```python
from build123d import *

# Parameters (mm, degrees)
SKETCH_W        = 142
SKETCH_H        = 67
PAD_DEPTH       = 25
THICKNESS_T     = 2.5
SKETCH001_R     = 4.3
SKETCH001_R_2   = 1.8
PAD001_DEPTH    = 5.5
FILLET_R        = 1
SKETCH002_W     = 32
SKETCH002_H     = 18.6
POCKET_DEPTH    = 5
SKETCH003_W     = 52
SKETCH003_H     = 20
POCKET001_DEPTH = 2.5
SKETCH006_R     = 1.8
POCKET002_DEPTH = 27.501
PAD005_DEPTH    = 2.5
FILLET001_R     = 2
CHAMFER001_SIZE = 1.2
FILLET002_R     = 2
CHAMFER002_SIZE = 1.2
POCKET003_DEPTH = 3
CHAMFER003_SIZE = 0.7


with BuildPart() as part:
    # Sketch → Pad (new body)
    with BuildSketch(Plane.XY):
        Rectangle(SKETCH_W, SKETCH_H)
    extrude(amount=PAD_DEPTH)

    # Thickness
    thickness_openings = [part.faces().sort_by_distance(p)[0] for p in [
        (0, 0, 25),
    ]]
    offset(amount=THICKNESS_T, openings=thickness_openings)

    # Sketch001 (on Face5 of Thickness) → Pad001 (join)
    with BuildSketch(Plane.XY):
        with Locations((-65, -27.5)):
            Circle(SKETCH001_R)
        with Locations((-65, -27.5)):
            Circle(SKETCH001_R_2, mode=Mode.SUBTRACT)
        with Locations((-65, 27.5)):
            Circle(SKETCH001_R)
        with Locations((-65, 27.5)):
            Circle(SKETCH001_R_2, mode=Mode.SUBTRACT)
        with Locations((-20, 27.5)):
            Circle(SKETCH001_R)
        with Locations((-20, 27.5)):
            Circle(SKETCH001_R_2, mode=Mode.SUBTRACT)
        with Locations((65, 27.5)):
            Circle(SKETCH001_R)
        with Locations((65, 27.5)):
            Circle(SKETCH001_R_2, mode=Mode.SUBTRACT)
        with Locations((65, -27.5)):
            Circle(SKETCH001_R)
        with Locations((65, -27.5)):
            Circle(SKETCH001_R_2, mode=Mode.SUBTRACT)
    extrude(amount=PAD001_DEPTH)

    # Fillet
    fillet_edges = [part.edges().sort_by_distance(p)[0] for p in [
        (-71, 33.5, 12.5),
        (71, 33.5, 12.5),
        (-71, -33.5, 12.5),
        (71, -33.5, 12.5),
    ]]
    fillet(fillet_edges, radius=FILLET_R)

    # Sketch002 (on Face19 of Fillet) → Pocket (cut)
    with BuildSketch(Plane(origin=(0, 36, 0), x_dir=(-1, 0, 0), z_dir=(0, 1, 0))):
        with Locations((-5.2475, 15.7)):
            Rectangle(SKETCH002_W, SKETCH002_H)
        with Locations((43.65, 15.7)):
            Rectangle(SKETCH002_W, SKETCH002_H)
        with BuildLine():
            ThreePointArc((-42.45, 25), (-47.8, 30.35), (-53.15, 25))
            Line((-53.15, 25), (-53.15, 9.6))
            ThreePointArc((-53.15, 9.6), (-47.8, 4.25), (-42.45, 9.6))
            Line((-42.45, 25), (-42.45, 9.6))
        make_face()
        with BuildLine():
            ThreePointArc((-25.95, 25), (-31.3, 30.35), (-36.65, 25))
            Line((-36.65, 25), (-36.65, 9.6))
            ThreePointArc((-36.65, 9.6), (-31.3, 4.25), (-25.95, 9.6))
            Line((-25.95, 25), (-25.95, 9.6))
        make_face()
    extrude(amount=-POCKET_DEPTH, mode=Mode.SUBTRACT)

    # Sketch003 (on Face35 of Pocket) → Pocket001 (cut)
    with BuildSketch(Plane.XZ.offset(36)):
        with Locations((-1.1, 15)):
            Rectangle(SKETCH003_W, SKETCH003_H)
    extrude(amount=-POCKET001_DEPTH, mode=Mode.SUBTRACT)

    # Sketch006 (on Face61 of Pocket001) → Pocket002 (cut, through all)
    with BuildSketch(Plane(origin=(0, 0, -2.5), x_dir=(1, 0, 0), z_dir=(0, 0, -1))):
        with Locations((-65, 27.5)):
            Circle(SKETCH006_R)
        with Locations((65, 27.5)):
            Circle(SKETCH006_R)
        with Locations((65, -27.5)):
            Circle(SKETCH006_R)
        with Locations((-20, -27.5)):
            Circle(SKETCH006_R)
        with Locations((-65, -27.5)):
            Circle(SKETCH006_R)
    extrude(amount=-POCKET002_DEPTH, mode=Mode.SUBTRACT)

    # Sketch008 (on Face32 of Pocket002) → Pad005 (join)
    with BuildSketch(Plane(origin=(0, 36, 0), x_dir=(-1, 0, 0), z_dir=(0, 1, 0))):
        with BuildLine():
            ThreePointArc((-42.45, 9.6), (-47.8, 14.95), (-53.15, 9.6))
            Line((-53.15, 9.6), (-53.15, 25))
            Line((-53.15, 25), (-42.45, 25))
            Line((-42.45, 25), (-42.45, 9.6))
        make_face()
        with BuildLine():
            ThreePointArc((-25.95, 9.6), (-31.3, 14.95), (-36.65, 9.6))
            Line((-36.65, 9.6), (-36.65, 25))
            Line((-36.65, 25), (-25.95, 25))
            Line((-25.95, 25), (-25.95, 9.6))
        make_face()
    extrude(amount=-PAD005_DEPTH)

    # Fillet001
    fillet001_edges = [part.edges().sort_by_distance(p)[0] for p in [
        (21.2475, 34.75, 6.4),
        (-10.7525, 34.75, 6.4),
        (-27.65, 34.75, 6.4),
        (-59.65, 34.75, 6.4),
    ]]
    fillet(fillet001_edges, radius=FILLET001_R)

    # Chamfer001
    chamfer001_edges = [part.edges().sort_by_distance(p)[0] for p in [
        (31.3, 36, 4.25),
        (47.8, 36, 4.25),
        (5.2475, 36, 6.4),
        (-43.65, 36, 6.4),
    ]]
    chamfer(chamfer001_edges, length=CHAMFER001_SIZE)

    # Fillet002
    fillet002_edges = [part.edges().sort_by_distance(p)[0] for p in [
        (24.9, -34.75, 5),
        (-27.1, -34.75, 5),
    ]]
    fillet(fillet002_edges, radius=FILLET002_R)

    # Chamfer002
    chamfer002_edges = [part.edges().sort_by_distance(p)[0] for p in [
        (-1.1, -36, 5),
    ]]
    chamfer(chamfer002_edges, length=CHAMFER002_SIZE)

    # Sketch010 (on Face14 of Chamfer002) → Pocket003 (cut)
    with BuildSketch(Plane.XY.offset(25)):
        with BuildLine():
            Line((-70, 33.7), (70, 33.7))
            ThreePointArc((71.2, 32.5), (70.848528, 33.348528), (70, 33.7))
            Line((71.2, 32.5), (71.2, -32.5))
            ThreePointArc((70, -33.7), (70.848528, -33.348528), (71.2, -32.5))
            Line((70, -33.7), (-70, -33.7))
            ThreePointArc((-71.2, -32.5), (-70.848528, -33.348528), (-70, -33.7))
            Line((-71.2, -32.5), (-71.2, 32.5))
            ThreePointArc((-70, 33.7), (-70.848528, 33.348528), (-71.2, 32.5))
        make_face()
    extrude(amount=-POCKET003_DEPTH, mode=Mode.SUBTRACT)

    # Chamfer003
    chamfer003_edges = [part.edges().sort_by_distance(p)[0] for p in [
        (-65.925, 36, 25),
        (-19.20125, 36, 25),
        (31.3, 36, 25),
    ]]
    chamfer(chamfer003_edges, length=CHAMFER003_SIZE)


solid = part.part
```
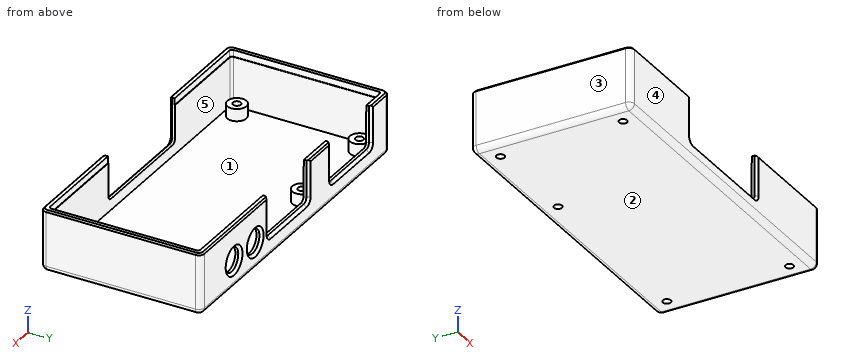
Check sheet for the modelled part. Datum: model origin and axes. Units: mm. Face numbers are marked on the shaded views. A direction names the side the tool comes from. Give positions to 0.01 mm unless a question says otherwise; leave off trailing zeros. Order: outer loops, then holes, each group sorted by start corner. A loop starts at its lowest first (then second) coordinate and runs counter-clockwise, first axis right, second up. Notation, with made-up numbers: M -23.75,-24.75 L -14.75,-24.75 A26 ccw -14.75,-5.75 Z; hole C 13.25,84 d9. An arc over 180 degrees is marked long. Answer in a Markdown table with one row per item. Add a question column.
Q1. Access from +Z, -Z, +X, -X, +Y, -Y to the whole of each face (thin tool, end or side, straight path). Record for the marked faces 1 and 2.
Q2. Sectioned sample at B-B, the plane x = 47.8. Record the boundary of the cut face in (y, z), and give its area (3 significant figures).
Q3. Sectioned sample at A-A, the plane y = -27.5. Count the separate pieces of the cut face and the enclosed holes in it, and give its area (3 significant figures).
Q4. Thickness scan on L1, parallel to Y at x = -65, z = 2; L2, parallel to X at y = -23.5, z = 21; L3, parallel to Y at x = 54, z = 20.5. Record the ranges inside material, lowest first.
Q5. Gauge pin test, flat ends, axial feed: pin 1 Ø0.6 at (y, z) = (34, 17) entering from +X; pin 2 Ø2.5 at (x, y) = (63.5, -29) entering from +Z; pin 3 Ø2 at (x, z) = (-10.5, 13) entering from -Y. Record the tip position at first contact, or that the pin passes through.
Q6. Release check for a two-part mould opening along Y. For the marked faces 3, 4 and 5 record: released by +Y, released by -Y, zero draft, split by the parting line, or undercut.
Verdict:
| question | item | result |
|---|---|---|
| 1 | face 1 | +Z |
| 1 | face 2 | -Z, +X, -X, +Y, -Y |
| 2 | outline | M -36,0 A2.5 ccw -33.5,-2.5 L 33.5,-2.5 A2.5 ccw 36,0 L 36,3.05 L 34.8,4.25 L 33.5,4.25 L 33.5,0 L -33.5,0 L -33.5,22 L -33.7,22 L -33.7,25 L -35.3,25 L -36,24.3 Z; M 33.5,14.95 L 34.8,14.95 L 36,16.15 L 36,24.3 L 35.3,25 L 33.7,25 L 33.7,22 L 33.5,22 Z |
| 2 | area | 272 mm² |
| 3 | separate pieces | 3 |
| 3 | enclosed holes | 0 |
| 3 | area | 525 mm² |
| 4 | L1 | -36 to -33.5, -31.8 to -29.3, -25.7 to -23.2, 23.2 to 25.7, 29.3 to 31.8, 33.5 to 36 |
| 4 | L2 | -73.5 to -71, 71 to 73.5 |
| 4 | L3 | -36 to -33.5, 33.5 to 36 |
| 5 | pin 1 | x = 73.49 |
| 5 | pin 2 | z = 5.5 |
| 5 | pin 3 | y = 33.5 |
| 6 | face 3 | zero draft |
| 6 | face 4 | released by -Y |
| 6 | face 5 | undercut |
